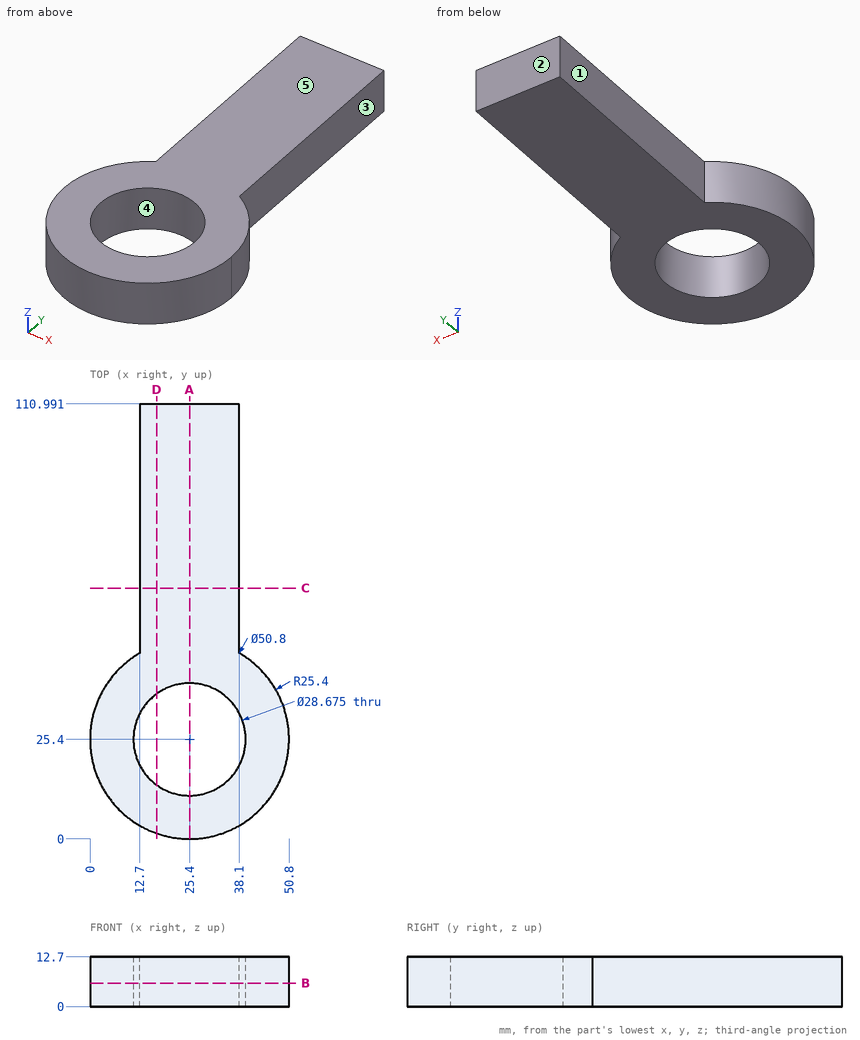
Answer from the drawing. Dimensions are ordinates in mm from the lowest x, y and z of the part. A direction names the side the tool comes from. Coordinates: 2 decimals unless noted, no trailing zeros. Loops run counter-clockwise (first coordinate to the right, second up) from the corner with the lowest first, then second, coordinate; pieces in that order, holes last. Notation, with made-up numbers: (50, 63.5) -> (102, 63.5) arc R24 ccw to (102, 74.5) -> close; hole circle Ø9 at (37.5, 40.5). An arc over 180 degrees is marked (long way). Answer in a Markdown table with one row per item.
Item 1: Each of these flat-tipped pins is pushed along its axis until it touches: P1, Ø1, axis at x = 37, z = 11, coming from the -Y side; P2, Ø4, axis at y = 84.5, z = 8.5, coming from the -X side; P3, Ø6.5, axis at y = 80, z = 5.5, coming from the +X side; P4, Ø23, axis at x = 25.4, y = 25.4, coming from the -Z side. Where does it stop, or does it pass through?
Returned:
| item | result |
|---|---|
| P1 | stops at y = 2.55 |
| P2 | stops at x = 12.7 |
| P3 | stops at x = 38.1 |
| P4 | passes through |
Item 2: A cutting plane is placed at A-A on x = 25.4. Determine the outline of the cut face in (y, z).
Returned:
| item | result |
|---|---|
| outline | (0, 0) -> (11.06, 0) -> (11.06, 12.7) -> (0, 12.7) -> close; (39.74, 0) -> (110.99, 0) -> (110.99, 12.7) -> (39.74, 12.7) -> close |
Item 3: A cutting plane is placed at B-B on z = 6. Determine the outline of the cut face in (x, y) (1 decimal), plus the area to 3 significant figures.
Returned:
| item | result |
|---|---|
| outline | (12.7, 47.4) arc R25.4 ccw (long way) to (38.1, 47.4) -> (38.1, 111) -> (12.7, 111) -> close; hole circle Ø28.7 at (25.4, 25.4) |
| area | 2,940 mm^2 |
Item 4: For a pull along X with two mould halves and no side action, classify the marked faces 3, 4 and 5 as released by +X, released by -X, zero draft, split by the parting line, or undercut.
Returned:
| item | result |
|---|---|
| face 3 | released by +X |
| face 4 | undercut |
| face 5 | zero draft |
Item 5: A cutting plane is placed at C-C on y = 64. Determine the outline of the cut face in (x, z).
Returned:
| item | result |
|---|---|
| outline | (12.7, 0) -> (38.1, 0) -> (38.1, 12.7) -> (12.7, 12.7) -> close |
Item 6: For the marked faces 1 and 2, determine the directions among +Z, -Z, +X, -X, +Y, -Y from which every point of the face is accessible in a straight line to the end or side of a thin tool.
Returned:
| item | result |
|---|---|
| face 1 | +Z, -Z, -X, +Y |
| face 2 | +Z, -Z, +X, -X, +Y |
Item 7: Straight lines are drawn through the part: line 1 along X through (y, z) = (25.4, 4.75); line 2 along Y through (x, z) = (25.4, 8.5); line 3 along X through (y, z) = (53.5, 9.5). For each, find the intervals that lie inside material, in ascending order. Write a range as [from, to].
Returned:
| item | result |
|---|---|
| line 1 | x = [0, 11.06], [39.74, 50.8] |
| line 2 | y = [0, 11.06], [39.74, 110.99] |
| line 3 | x = [12.7, 38.1] |
Item 8: A cutting plane is placed at D-D on x = 17. Determine the outline of the cut face in (y, z), plus the area to 3 significant figures.
Returned:
| item | result |
|---|---|
| outline | (1.43, 0) -> (13.78, 0) -> (13.78, 12.7) -> (1.43, 12.7) -> close; (37.02, 0) -> (110.99, 0) -> (110.99, 12.7) -> (37.02, 12.7) -> close |
| area | 1,100 mm^2 |
